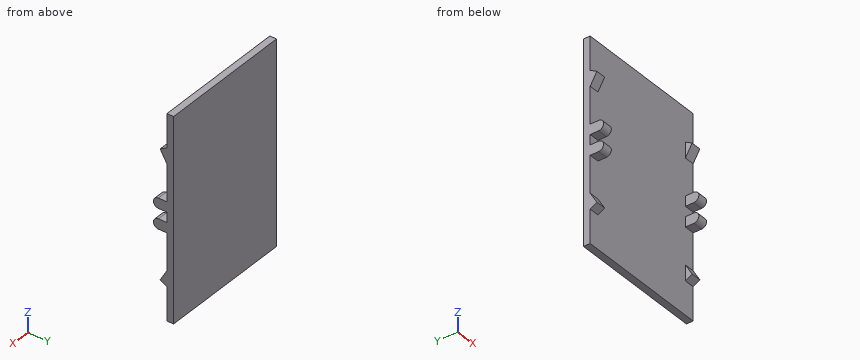
```python
from build123d import *

# Parameters (mm, degrees)
SKETCH1_W            = 400
SKETCH1_H            = 600
BOSS_EXTRUDE1_DEPTH  = 20
BOSS_EXTRUDE2_DEPTH  = 30
MIRROR2_COPY_1_DEPTH = 30
BOSS_EXTRUDE3_DEPTH  = 30
MIRROR4_COPY_1_DEPTH = 30


with BuildPart() as part:
    # Sketch1 → Boss-Extrude1 (new body)
    with BuildSketch(Plane(origin=(0, 0, 0), x_dir=(1, 0, 0), z_dir=(0, 1, 0))):
        Rectangle(SKETCH1_W, SKETCH1_H)
    extrude(amount=BOSS_EXTRUDE1_DEPTH)

    # Sketch3 → Boss-Extrude2 (add)
    with BuildSketch(Plane(origin=(200, 0, 0), x_dir=(0, 0, -1), z_dir=(1, 0, 0))):
        with BuildLine():
            Line((-45, -25), (-45, 0))
            Line((-45, 0), (-15, 0))
            Line((-15, 0), (-15, -25))
            ThreePointArc((-15, -25), (-30, -40), (-45, -25))
        make_face()
    boss_extrude2 = extrude(amount=-BOSS_EXTRUDE2_DEPTH)

    # Mirror1: Boss-Extrude2 across plane
    add(boss_extrude2.mirror(Plane.XY))

    # Mirror2: Boss-Extrude2 across plane
    add(boss_extrude2.mirror(Plane(origin=(0, 0, 0), x_dir=(0, 0, 1), z_dir=(1, 0, 0))))

    # Mirror2 copy 1 sketch → Mirror2 copy 1 (add)
    with BuildSketch(Plane.ZY.offset(200)):
        with BuildLine():
            Line((-45, -25), (-45, 0))
            Line((-45, 0), (-15, 0))
            Line((-15, 0), (-15, -25))
            ThreePointArc((-15, -25), (-30, -40), (-45, -25))
        make_face()
    extrude(amount=-MIRROR2_COPY_1_DEPTH)

    # Sketch4 → Boss-Extrude3 (add)
    with BuildSketch(Plane(origin=(200, 0, 0), x_dir=(0, 0, -1), z_dir=(1, 0, 0))):
        Polygon((-154.598033597, 0), (-189.239049749, -20), (-200.786055132, 0), align=None)
    boss_extrude3 = extrude(amount=-BOSS_EXTRUDE3_DEPTH)

    # Mirror3: Boss-Extrude3 across plane
    add(boss_extrude3.mirror(Plane(origin=(0, 0, 0), x_dir=(0, 0, 1), z_dir=(1, 0, 0))))

    # Mirror4: Boss-Extrude3 across plane
    add(boss_extrude3.mirror(Plane.XY))

    # Mirror4 copy 1 sketch → Mirror4 copy 1 (add)
    with BuildSketch(Plane.ZY.offset(200)):
        Polygon((-154.598033597, 0), (-189.239049749, -20), (-200.786055132, 0), align=None)
    extrude(amount=-MIRROR4_COPY_1_DEPTH)


solid = part.part
```
Part model, mm, in its own coordinate system. Round coordinates to 2 decimals unless told otherwise and drop trailing zeros. Loops run counter-clockwise (first coordinate to the right, second up) from the corner with the lowest first, then second, coordinate; pieces in that order, holes last.
Item 1: Drill centre lines: line 1 (X direction, y = -0.5, z = -41); line 2 (Y direction, x = -146, z = -46.5); line 3 (Y direction, x = -174.5, z = -33). Where is each one in solid material? Low to high.
Item 2: Cut at A-A, the plane z = 30. Give the cut face in (x, y).
Item 3: Cut at B-B, the plane y = -8. State how many separate pieces and enclosed holes the cut face has, then the cut area to 3 significant figures.
Item 4: Cut at D-D, the plane z = -171. Give the cut face in (x, y).
Item 5: Cut at C-C, the plane x = -135. Give the cut face in (y, z).
Item 6: Drop flat-ended pins along their axis: P1, Ø20, axis at x = -188, y = -17.5, coming from the -Z side; P2, Ø20, axis at x = -181.5, y = -13.5, coming from the -Z side; P3, Ø12.5, axis at x = 181.5, y = -18, coming from the -Z side. Give the stop position or say it passes through.
A:
1. line 1: x = -200 to -170, 170 to 200
1. line 2: y = 0 to 20
1. line 3: y = -39.7 to 20
2. outline: (-200, -40) - (-170, -40) - (-170, 0) - (170, 0) - (170, -40) - (200, -40) - (200, 20) - (-200, 20) - close
3. separate pieces: 8
3. enclosed holes: 0
3. area: 6,930 mm2
4. outline: (-200, -9.47) - (-170, -9.47) - (-170, 0) - (170, 0) - (170, -9.47) - (200, -9.47) - (200, 20) - (-200, 20) - close
5. outline: (0, -300) - (20, -300) - (20, 300) - (0, 300) - close
6. P1: stops at z = -196.46
6. P2: stops at z = -198.77
6. P3: stops at z = -194
